```python
from build123d import *

# Parameters (mm, degrees)
ESBO_O2_W                = 2
ESBO_O2_H                = 0.5
RESSALTO_EXTRUS_O1_DEPTH = 6


with BuildPart() as part:
    # Esboço1 → Revolução1 (revolve)
    with BuildSketch(Plane.XY):
        Polygon((0, 22.689764513), (4, 22.689764513), (4, 19), (5.891304348, 19), (7, 18.5), (7, 17), (6.5, 17), (6.5, 10), (5.5, 10), (5.5, 6), (3.5, 6), (3.5, 0), (0, 0), align=None)
    revolve(axis=Axis((0, 0, 0), (0, 1, 0)))

    # Esboço2 → Ressalto-extrusão1 (add)
    with BuildSketch(Plane.XZ):
        with Locations((0, -1.75)):
            Rectangle(ESBO_O2_W, ESBO_O2_H)
        with Locations((0, 1.75)):
            Rectangle(ESBO_O2_W, ESBO_O2_H)
    extrude(amount=RESSALTO_EXTRUS_O1_DEPTH)


solid = part.part
```
For this review, take the finished solid that the model builds, in its own axes (mm). A direction names the side the tool comes from. Give positions to 0.01 mm unless a question says otherwise; leave off trailing zeros. Order: outer loops, then holes, each group sorted by start corner. A loop starts at its lowest first (then second) coordinate and runs counter-clockwise, first axis right, second up.
1) For faces 4 (the face through (-0.867, 20.819, 3.905)), 5 (the face through (0, -3, -2)), 6 (the face through (0, -3, 2)), 7 (the face through (0, -3, 1.5)), list the 3-axis set-ups (+Z, -Z, +X, -X, +Y, -Y) from which the entire face can be reached by the end or side of a thin tool; tool diameter is ignored.
2) The part is to be moulded in two halves that separate along Z. For faces 1 (the face through (0, 22.69, 0)), 2 (the face through (3.233, 2.958, 1.341)), 3 (the face through (0, -3, -1.5)), say which applies: released by +Z, released by -Z, zero draft, split by the parting line, or undercut.
3) Wall thickness on line 1 (Y direction, x = 3, z = 4); line 2 (Y direction, x = 1.25, z = -0.5); line 3 (Z direction, x = 0.25, y = 16.5): over which ranges is each line inside the solid? List them lowest first.
4) Take a section at A-A (z = 0). Give the boundary of the cut face in (x, y).
5) Take a section at C-C (y = 13). Give the boundary of the cut face in (x, z).
6) Insertion check: pin 1 (2 mm diameter, centred on x = 1.5, z = 5, fed in from -Y); pin 2 (2 mm diameter, centred on x = 0, y = -2, fed in from -Z); pin 3 (2 mm diameter, centred on x = -0.5, y = -3, fed in from +Z). Each pin has a flat end and moves straight along its axis. Give the tip position at first contact, or say it passes through.
Derived:
1. face 4: +Y
1. face 5: -Z, +X, -X, -Y
1. face 6: +Z, +X, -X, -Y
1. face 7: +X, -X, -Y
2. face 1: zero draft
2. face 2: split by the parting line
2. face 3: undercut
3. line 1: y = 6 to 19
3. line 2: y = 0 to 22.69
3. line 3: z = -6.5 to 6.5
4. outline: (-7, 17) - (-6.5, 17) - (-6.5, 10) - (-5.5, 10) - (-5.5, 6) - (-3.5, 6) - (-3.5, 0) - (3.5, 0) - (3.5, 6) - (5.5, 6) - (5.5, 10) - (6.5, 10) - (6.5, 17) - (7, 17) - (7, 18.5) - (5.89, 19) - (4, 19) - (4, 22.69) - (-4, 22.69) - (-4, 19) - (-5.89, 19) - (-7, 18.5) - close
5. outline: circle Ø13 at (0, 0)
6. pin 1: stops at y = 6
6. pin 2: stops at z = -2
6. pin 3: stops at z = 2
